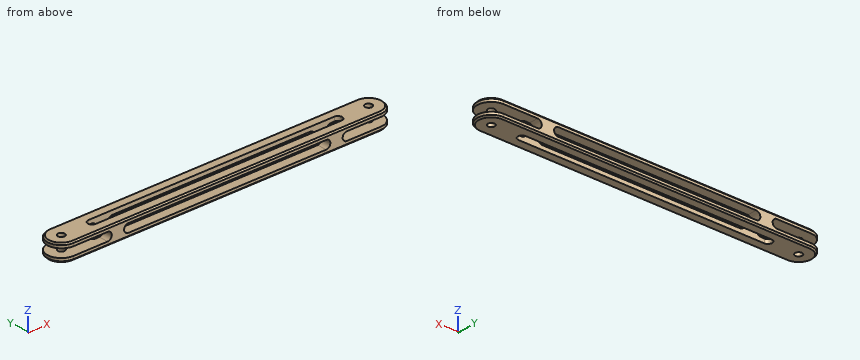
```python
from build123d import *

# Parameters (mm, degrees)
BOSS_EXTRUDE1_DEPTH = 6
CUT_EXTRUDE1_DEPTH  = 51
SKETCH4_R           = 2.5
CUT_EXTRUDE2_DEPTH  = 102
CHAMFER1_SIZE       = 1


with BuildPart() as part:
    # Sketch2 → Boss-Extrude1 (new, symmetric)
    with BuildSketch(Plane.XY):
        with BuildLine():
            Line((-112.5, 10), (112.5, 10))
            ThreePointArc((112.5, 10), (122.5, 0), (112.5, -10))
            Line((112.5, -10), (-112.5, -10))
            ThreePointArc((-112.5, -10), (-122.5, 0), (-112.5, 10))
        make_face()
    extrude(amount=BOSS_EXTRUDE1_DEPTH, both=True)

    # Sketch3 → Cut-Extrude1 (cut, symmetric)
    with BuildSketch(Plane(origin=(0, 0, 0), x_dir=(1, 0, 0), z_dir=(0, 1, 0))):
        with BuildLine():
            Line((-72.5, 3), (72.5, 3))
            ThreePointArc((72.5, 3), (75.5, 0), (72.5, -3))
            Line((72.5, -3), (-72.5, -3))
            ThreePointArc((-72.5, -3), (-75.5, 0), (-72.5, 3))
        make_face()
        with BuildLine():
            Line((157.5, -3), (87.5, -3))
            ThreePointArc((87.5, -3), (84.5, 0), (87.5, 3))
            Line((87.5, 3), (157.5, 3))
            ThreePointArc((157.5, 3), (160.5, 0), (157.5, -3))
        make_face()
        with BuildLine():
            Line((-157.5, -3), (-87.5, -3))
            ThreePointArc((-87.5, -3), (-84.5, 0), (-87.5, 3))
            Line((-87.5, 3), (-157.5, 3))
            ThreePointArc((-157.5, 3), (-160.5, 0), (-157.5, -3))
        make_face()
    extrude(amount=CUT_EXTRUDE1_DEPTH, both=True, mode=Mode.SUBTRACT)

    # Sketch4 → Cut-Extrude2 (cut)
    with BuildSketch(Plane.XY.offset(6)):
        with Locations((112.5, 0)):
            Circle(SKETCH4_R)
        with Locations((-112.5, 0)):
            Circle(SKETCH4_R)
        with BuildLine():
            Line((-90, 3), (90, 3))
            ThreePointArc((90, 3), (93, 0), (90, -3))
            Line((90, -3), (-90, -3))
            ThreePointArc((-90, -3), (-93, 0), (-90, 3))
        make_face()
    extrude(amount=-CUT_EXTRUDE2_DEPTH, mode=Mode.SUBTRACT)

    # Chamfer1
    chamfer1_edges = [part.edges().sort_by_distance(p)[0] for p in [
        (122.5, 0, -6),
        (0, 10, -6),
        (-122.5, 0, -6),
        (0, 10, 6),
        (122.5, 0, 6),
        (0, -10, 6),
        (-122.5, 0, 6),
        (0, -10, -6),
    ]]
    chamfer(chamfer1_edges, length=CHAMFER1_SIZE)


solid = part.part
```
Can you work these out from the model? Positions are in its coordinate system, mm. Coordinates: 2 decimals unless noted, no trailing zeros. Loops run counter-clockwise (first coordinate to the right, second up) from the corner with the lowest first, then second, coordinate; pieces in that order, holes last. Notation, with made-up numbers: (75, 63) - (110, 63) arc R15 ccw to (110, 89) - close; hole circle Ø11 at (21.25, 35.5). An arc over 180 degrees is marked (long way). Use a Markdown table: item, result.
Item 1: I want a section at C-C on y = 0. Give the number of separate pieces and of enclosed holes in the cut face, and give its area (3 significant figures).
Numbers:
| item | result |
|---|---|
| separate pieces | 8 |
| enclosed holes | 0 |
| area | 292 mm2 |
Item 2: Will these pins go through, and if not, where does the flat tip stop? pin 1 (3.5 mm diameter, centred on x = 24, z = 0, fed in from +Y); pin 2 (6 mm diameter, centred on y = 6.5, z = 1, fed in from -X); pin 3 (6 mm diameter, centred on y = -5, z = -4, fed in from +X).
Numbers:
| item | result |
|---|---|
| pin 1 | passes through |
| pin 2 | stops at x = -121.55 |
| pin 3 | stops at x = 122.3 |
Item 3: I want a section at A-A on x = 59.5. Please give me the cut outline in (y, z), and give its area (3 significant figures).
Numbers:
| item | result |
|---|---|
| outline | (-10, -5) - (-9, -6) - (-3, -6) - (-3, -3) - (-10, -3) - close; (-10, 3) - (-3, 3) - (-3, 6) - (-9, 6) - (-10, 5) - close; (3, -6) - (9, -6) - (10, -5) - (10, -3) - (3, -3) - close; (3, 3) - (10, 3) - (10, 5) - (9, 6) - (3, 6) - close |
| area | 82.0 mm2 |
Item 4: If I drill on probe 1 along X at (y, z) = (-5, -0.25); probe 2 along Y at (x, z) = (-112.5, -4.3); probe 3 along Z at (x, y) = (-51.5, -8.75), over which ranges is the centre line in solid material (lowest first)? Write a range as from..to.
Numbers:
| item | result |
|---|---|
| probe 1 | x = -84.51..-75.49, 75.49..84.51 |
| probe 2 | y = -10..-2.5, 2.5..10 |
| probe 3 | z = -6..-3, 3..6 |
Item 5: I want a section at B-B on z = 0.5. Please give me the cut outline in (x, y), and give its area (3 significant figures).
Numbers:
| item | result |
|---|---|
| outline | (-84.54, -10) - (-75.46, -10) - (-75.46, -3) - (-84.54, -3) - close; (-84.54, 3) - (-75.46, 3) - (-75.46, 10) - (-84.54, 10) - close; (75.46, -10) - (84.54, -10) - (84.54, -3) - (75.46, -3) - close; (75.46, 3) - (84.54, 3) - (84.54, 10) - (75.46, 10) - close |
| area | 254 mm2 |
